Geometry check sheet. Reference: the model listing, model coordinates, mm. Face numbers are marked on the shaded views. A direction names the side the tool comes from. Round coordinates to 2 decimals unless told otherwise and drop trailing zeros. Write each loop counter-clockwise with the first axis right and the second up, starting at its lowest first coordinate (ties: lowest second). Pieces come first, ordered by that corner, then holes. Notation, with made-up numbers: (33, 55) -> (78, 55) arc R23 ccw to (78, 79) -> close; hole circle Ø3 at (1, -30). An arc over 180 degrees is marked (long way). Return JSON: item names as keys, results as strings. Group by question number.
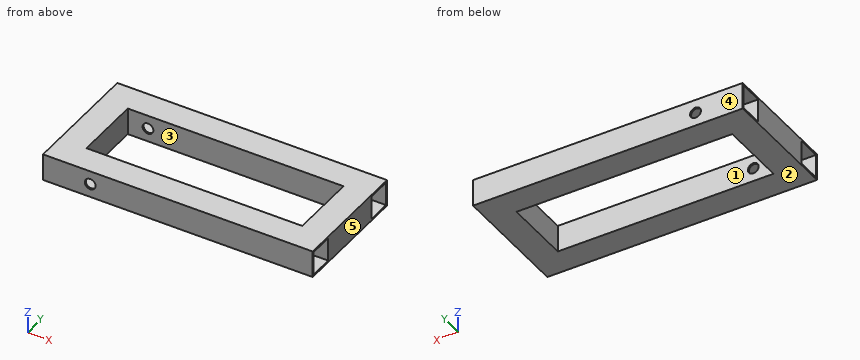
from build123d import *

# Parameters (mm, degrees)
F0_W     = 20
F0_H     = 20
F0_W_2   = 17.5
F0_H_2   = 17.5
F1_DEPTH = 200
F2_W     = 20
F2_H     = 20
F2_W_2   = 17.5
F2_H_2   = 17.5
F3_DEPTH = 50
F4_R     = 4
F5_DEPTH = 20.001


with BuildPart() as f1:
    # F0 (on Right) → F1 (new body)
    with BuildSketch(Plane.YZ):
        with Locations((10, 10)):
            Rectangle(F0_W, F0_H)
        with Locations((10, 10)):
            Rectangle(F0_W_2, F0_H_2, mode=Mode.SUBTRACT)
    extrude(amount=F1_DEPTH)

    # F2 (on face) → F3 (join)
    with BuildSketch(Plane.XZ):
        with Locations((10, 10)):
            Rectangle(F2_W, F2_H)
        with Locations((10, 10)):
            Rectangle(F2_W_2, F2_H_2, mode=Mode.SUBTRACT)
        with Locations((190, 10)):
            Rectangle(F2_W, F2_H)
        with Locations((190, 10)):
            Rectangle(F2_W_2, F2_H_2, mode=Mode.SUBTRACT)
    extrude(amount=F3_DEPTH)

    # F4 (on face) → F5 (cut, through all)
    with BuildSketch(Plane.XZ):
        with Locations((35, 10)):
            Circle(F4_R)
    extrude(amount=-F5_DEPTH, mode=Mode.SUBTRACT)

    # F8: F1 across plane


with BuildPart() as f1_1:
    add(f1.part)
    add(f1.part.mirror(Plane.XZ.offset(25)))


solid = f1_1.part
1) Sectioned sample at B-B on x = 100.5. Enter the section's corners in (y, z), and give its area (4 significant figures).
2) Sectioned sample at C-C on y = 13.5. Enter the section's corners in (x, z), and give its area (3 significant figures).
3) Tool access check on the marked faces 1 and 2. Record the directions out of +Z, -Z, +X, -X, +Y, -Y that give a thin tool (end or side, any length) a straight path to the whole face; none if there is none.
4) Mould release check, pull along Y, two halves, no side actions. Record for the marked faces 3, 4 and 5: +Y half, -Y half, draft (parallel to the pull), parting line (faces both ways), or undercut.
5) Go/stop test with a flat-tipped pin: P1, Ø9, axis at x = 35, z = 10, coming from the +Y side. Record where the tip stops, or that it passes through.
6) Sectioned sample at D-D on z = 16.5. Enter the section's corners in (x, y).
7) Sectioned sample at A-A on y = -23.5. Enter the section's corners in (x, z).
8) Material ranges on probe 1 along Y at (x, z) = (9, 11); probe 2 along X at (y, z) = (-38, 10); probe 3 along Z at (x, y) = (35, 19.3), recorded low to high. Write a range as [from, to].
Evaluation:
{
 "1": {"outline": "(-70, 0) -> (-50, 0) -> (-50, 20) -> (-70, 20) -> close; (0, 0) -> (20, 0) -> (20, 20) -> (0, 20) -> close; hole (-68.75, 1.25) -> (-51.25, 1.25) -> (-51.25, 18.75) -> (-68.75, 18.75) -> close; hole (1.25, 1.25) -> (18.75, 1.25) -> (18.75, 18.75) -> (1.25, 18.75) -> close", "area": "187.5 mm2"},
 "2": {"outline": "(0, 0) -> (200, 0) -> (200, 1.25) -> (0, 1.25) -> close; (0, 18.75) -> (200, 18.75) -> (200, 20) -> (0, 20) -> close", "area": "500 mm2"},
 "3": {"face 1": "+Z, -Z", "face 2": "-Z, +X, -X, +Y, -Y"},
 "4": {"face 3": "undercut", "face 4": "+Y half", "face 5": "draft"},
 "5": {"P1": "stops at y = 20"},
 "6": {"outline": "(0, -70) -> (200, -70) -> (200, -68.75) -> (0, -68.75) -> close; (0, -51.25) -> (200, -51.25) -> (200, 1.25) -> (0, 1.25) -> close; (0, 18.75) -> (200, 18.75) -> (200, 20) -> (0, 20) -> close; hole (1.25, -50) -> (18.75, -50) -> (18.75, 0) -> (1.25, 0) -> close; hole (20, -50) -> (180, -50) -> (180, 0) -> (20, 0) -> close; hole (181.25, -50) -> (198.75, -50) -> (198.75, 0) -> (181.25, 0) -> close"},
 "7": {"outline": "(0, 0) -> (20, 0) -> (20, 20) -> (0, 20) -> close; (180, 0) -> (200, 0) -> (200, 20) -> (180, 20) -> close; hole (1.25, 1.25) -> (18.75, 1.25) -> (18.75, 18.75) -> (1.25, 18.75) -> close; hole (181.25, 1.25) -> (198.75, 1.25) -> (198.75, 18.75) -> (181.25, 18.75) -> close"},
 "8": {"probe 1": "y = [-70, -68.75], [-51.25, -50], [0, 1.25], [18.75, 20]", "probe 2": "x = [0, 1.25], [18.75, 20], [180, 181.25], [198.75, 200]", "probe 3": "z = [0, 6], [14, 20]"}
}
